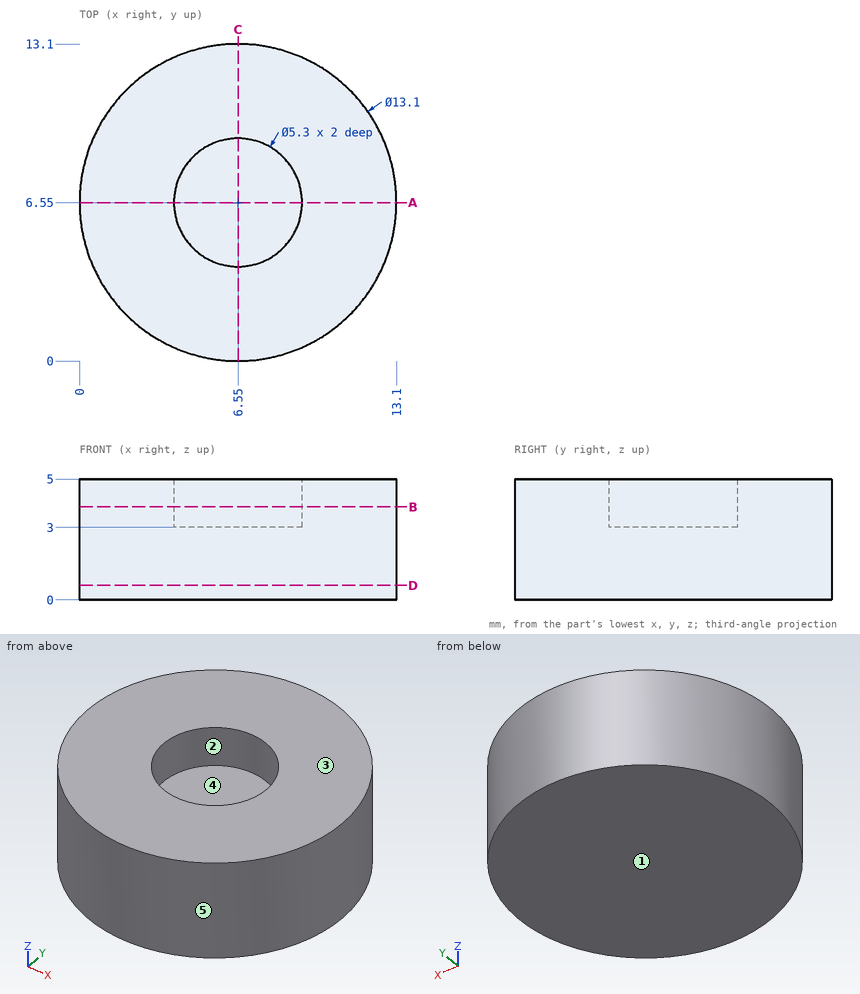
Input: dimensioned drawing with shaded views. Units: mm. Origin: part minimum x, y, z. A direction names the side the tool comes from. Give positions to 0.01 mm unless a question says otherwise; leave off trailing zeros. Order: outer loops, then holes, each group sorted by start corner. A loop starts at its lowest first (then second) coordinate and runs counter-clockwise, first axis right, second up. Notation, with made-up numbers: (-2, 76.5) -> (39, 76.5) arc R18 ccw to (39, 106.5) -> close; hole circle Ø11 at (2, 13). An arc over 180 degrees is marked (long way). Answer as a JSON object with one key per item and string values.
Q1. Access query for the marked faces 1 and 2. Directions: +Z, -Z, +X, -X, +Y, -Y. A direction counts if a zero-diameter tool reaches every point of the face in a straight line with its end or side. Return the directions, or none.
Entries:
{"face 1": "-Z, +X, -X, +Y, -Y", "face 2": "+Z"}
Q2. Draft query along X for the marked faces 3, 4 and 5. Return one class per face: released by +X, released by -X, zero draft, split by the parting line, or undercut.
Entries:
{"face 3": "zero draft", "face 4": "undercut", "face 5": "split by the parting line"}
Q3. Material intervals for probe 1 along Y at (x, z) = (6.5, 4.1); probe 2 along Z at (x, y) = (8.25, 7.25), sorted ascending.
Entries:
{"probe 1": "y = 0 to 3.9, 9.2 to 13.1", "probe 2": "z = 0 to 3"}
Q4. Section A-A (y = 6.55). Output: boundary loops of the cut face in (x, z), plus the area to 3 significant figures.
Entries:
{"outline": "(0, 0) -> (13.1, 0) -> (13.1, 5) -> (9.2, 5) -> (9.2, 3) -> (3.9, 3) -> (3.9, 5) -> (0, 5) -> close", "area": "54.9 mm^2"}
Q5. Section D-D (z = 0.6). Output: boundary loops of the cut face in (x, y), plus the area to 3 significant figures.
Entries:
{"outline": "circle Ø13.1 at (6.55, 6.55)", "area": "135 mm^2"}
Q6. First-contact query: pin 1 (6 mm diameter, centred on x = 7, y = 7, fed in from +Z). Flat tip, straight axial feed; report the tip coordinate or a pass-through.
Entries:
{"pin 1": "stops at z = 5"}
Q7. Section B-B (z = 3.85). Output: boundary loops of the cut face in (x, y), plus the area to 3 significant figures.
Entries:
{"outline": "circle Ø13.1 at (6.55, 6.55); hole circle Ø5.3 at (6.55, 6.55)", "area": "113 mm^2"}
